Check sheet for the modelled part. Datum: model origin and axes. Units: mm. Give positions to 0.01 mm unless a question says otherwise; leave off trailing zeros. Loops run counter-clockwise (first coordinate to the right, second up) from the corner with the lowest first, then second, coordinate; pieces in that order, holes last. Notation, with made-up numbers: (59.25, 4) -> (79.25, 4) arc R30 ccw to (79.25, 37) -> close; hole circle Ø8 at (19, 3). An arc over 180 degrees is marked (long way). Answer as CSV lines item,"result". Start each with the question number.
(1) Material ranges on line 1 (Y direction, x = 15, z = 0.2); line 2 (X direction, y = 15, z = 0.2); line 3 (Y direction, x = 13.5, z = 0.2), recorded low to high. Write a range as from..to.
(2) Section check D-D on y = 10. Enter the section's corners in (x, z), plus the area to 3 significant figures.
(3) Section check A-A on y = 18.5. Enter the section's corners in (x, z), plus the area to 3 significant figures.
(4) Section check C-C on z = 0.15. Enter the section's corners in (x, y) (3 decimals).
(5) Section check B-B on x = 17.5. Enter the section's corners in (y, z).
from build123d import *

# Parameters (mm, degrees)
BOSS_EXTRUDE1_DEPTH = 0.254
SKETCH2_R           = 4.699
CUT_EXTRUDE1_DEPTH  = 1.254
SKETCH3_W           = 2.54
SKETCH3_H           = 0.635
CUT_EXTRUDE2_DEPTH  = 1.254
SKETCH5_OUTSIDE_W   = 121.447
SKETCH5_OUTSIDE_H   = 109.618
CUT_EXTRUDE5_DEPTH  = 1.254


with BuildPart() as part:
    # Sketch1 → Boss-Extrude1 (new body)
    with BuildSketch(Plane.XY):
        with BuildLine():
            Line((67.21146711, 76.191723231), (8.696654013, 17.676910134))
            Line((8.696654013, 17.676910134), (7.228954972, 14.133571205))
            ThreePointArc((7.228954972, 14.133571205), (14.666587579, 6.075099489), (15.105587123, -4.88230096))
            Line((15.105587123, -4.88230096), (18.648926052, -6.35))
            Line((18.648926052, -6.35), (101.401368334, -6.35))
            ThreePointArc((101.401368334, -6.35), (93.866160503, 38.880636728), (67.21146711, 76.191723231))
        make_face()
        with BuildLine():
            Line((88.672924278, 6.35), (27.86051193, 6.35))
            ThreePointArc((27.86051193, 6.35), (26.399857642, 10.93517908), (24.190484974, 15.210228852))
            Line((24.190484974, 15.210228852), (67.191354125, 58.211098004))
            ThreePointArc((67.191354125, 58.211098004), (82.13289044, 34.020557137), (88.672924278, 6.35))
        make_face(mode=Mode.SUBTRACT)
    extrude(amount=BOSS_EXTRUDE1_DEPTH)

    # Sketch2 → Cut-Extrude1 (cut, through all)
    with BuildSketch(Plane.XY.offset(0.254)):
        with Locations((22.225, 0)):
            Circle(SKETCH2_R)
        with Locations((36.195, 0)):
            Circle(SKETCH2_R)
        with Locations((61.722, 0)):
            Circle(SKETCH2_R)
        with Locations((75.692, 0)):
            Circle(SKETCH2_R)
        with Locations((95.25, 0)):
            Circle(SKETCH2_R)
        with Locations((15.715448212, 15.715448212)):
            Circle(SKETCH2_R)
        with Locations((25.593729945, 25.593729945)):
            Circle(SKETCH2_R)
        with Locations((43.644044748, 43.644044748)):
            Circle(SKETCH2_R)
        with Locations((53.522326482, 53.522326482)):
            Circle(SKETCH2_R)
        with Locations((92.004434954, 24.652514046)):
            Circle(SKETCH2_R)
        with Locations((82.48891971, 47.625)):
            Circle(SKETCH2_R)
        with Locations((67.351920908, 67.351920908)):
            Circle(SKETCH2_R)
    extrude(amount=-CUT_EXTRUDE1_DEPTH, mode=Mode.SUBTRACT)

    # Sketch3 → Cut-Extrude2 (cut, through all)
    with BuildSketch(Plane.XY.offset(0.254)):
        Polygon((15.266435406, 24.246691527), (17.06248663, 26.042742751), (17.511499436, 25.593729945), (15.715448212, 23.797678721), align=None)
        Polygon((44.991083167, 53.971339288), (43.195031942, 52.175288063), (43.644044748, 51.726275257), (45.440095973, 53.522326482), align=None)
        with Locations((29.21, -6.0325)):
            Rectangle(SKETCH3_W, SKETCH3_H)
        with Locations((68.707, -6.0325)):
            Rectangle(SKETCH3_W, SKETCH3_H)
        Polygon((29.230733674, 38.210989795), (31.026784898, 40.007041019), (31.475797704, 39.558028213), (29.67974648, 37.761976989), align=None)
        Polygon((56.845021246, 65.825277367), (55.048970022, 64.029226143), (55.497982828, 63.580213337), (57.294034052, 65.376264561), align=None)
        with Locations((48.9585, -6.0325)):
            Rectangle(SKETCH3_W, SKETCH3_H)
        with Locations((85.471, -6.0325)):
            Rectangle(SKETCH3_W, SKETCH3_H)
        Polygon((99.935462164, 14.437711971), (100.266998693, 11.919442024), (101.526133667, 12.085210288), (101.194597138, 14.603480236), align=None)
        Polygon((93.765504959, 37.464305742), (94.938831965, 37.950313702), (93.966816047, 40.296967714), (92.793489041, 39.810959755), align=None)
        Polygon((79.327792988, 62.471156422), (80.874047017, 60.456038938), (81.88160576, 61.229165953), (80.33535173, 63.244283437), align=None)
        Polygon((13.593916116, 7.005422516), (14.565932035, 4.658768503), (15.739259041, 5.144776462), (14.767243123, 7.491430475), align=None)
    extrude(amount=-CUT_EXTRUDE2_DEPTH, mode=Mode.SUBTRACT)

    # Sketch5 outside → Cut-Extrude5 (cut, through all)
    with BuildSketch(Plane.XY.offset(0.254)):
        with Locations((54.4145, 34.921)):
            Rectangle(SKETCH5_OUTSIDE_W, SKETCH5_OUTSIDE_H)
        Polygon((8.194751981, 4.769015505), (26.967984082, 12.545142851), (12.599574288, 26.913552645), (-0.675105435, 13.638872921), align=None, mode=Mode.SUBTRACT)
    extrude(amount=-CUT_EXTRUDE5_DEPTH, mode=Mode.SUBTRACT)


solid = part.part
Working result:
1,line 1,"y = 7.59..11.07, 20.36..23.98"
1,line 2,"x = 7.59..11.07, 20.36..24.32"
1,line 3,"y = 8.35..11.57, 19.86..22.48"
2,outline,"(12.33, 0) -> (20.82, 0) -> (20.82, 0.25) -> (12.33, 0.25) -> close"
2,area,"2.16 mm^2"
3,outline,"(9.52, 0) -> (11.93, 0) -> (11.93, 0.25) -> (9.52, 0.25) -> close; (19.5, 0) -> (21.01, 0) -> (21.01, 0.25) -> (19.5, 0.25) -> close"
3,area,"0.996 mm^2"
4,outline,"(7.229, 14.134) arc R15.875 cw to (14.134, 7.229) -> (25.888, 12.098) arc R28.575 ccw to (24.19, 15.21) -> (24.247, 15.266) -> (15.266, 24.247) -> (8.697, 17.677) -> close; hole circle Ø9.398 at (15.715, 15.715)"
5,outline,"(8.62, 0) -> (11.37, 0) -> (11.37, 0.25) -> (8.62, 0.25) -> close; (20.06, 0) -> (22.01, 0) -> (22.01, 0.25) -> (20.06, 0.25) -> close"
